Source: CAD feature listing. Evaluate the final solid. Frame: model axes, mm. Face numbers are marked on the shaded views. A direction names the side the tool comes from. Give positions to 0.01 mm unless a question says otherwise; leave off trailing zeros. Order: outer loops, then holes, each group sorted by start corner. A loop starts at its lowest first (then second) coordinate and runs counter-clockwise, first axis right, second up. Notation, with made-up numbers: M 12,45.25 L 57,45.25 A19 cw 57,55.25 Z; hole C -32.75,67 d5. An arc over 180 degrees is marked long. Return JSON: item names as keys, results as strings.
from build123d import *

# Parameters (mm, degrees)
CONE_ROLL_ANGLE        = 90
CYLINDER_R             = 1
CYLINDER_DEPTH         = 3
CYLINDER_ROLL_ANGLE    = 90
CYLINDER005_R          = 3.5
CYLINDER005_DEPTH      = 3
CYLINDER005_ROLL_ANGLE = 90
BOX_W                  = 1
BOX_H                  = 10
BOX_DEPTH              = 10
BOX002_W               = 13
BOX002_H               = 5
BOX002_DEPTH           = 13
CYLINDER002_R          = 2.4
CYLINDER002_DEPTH      = 13
CYLINDER002_ROLL_ANGLE = 90


with BuildPart() as screw_guide:
    # Cone → Cone (revolve)
    with BuildSketch(Plane.XZ):
        Polygon((0, 0), (0.5, 0), (1.5, 7), (0, 7), align=None)
    revolve(axis=Axis((0, 0, 0), (0, 0, 1)))


with BuildPart() as screw_guide_1:
    # Cone roll: moved
    add(screw_guide.part.rotate(Axis((0, 0, 0), (1, 0, 0)), CONE_ROLL_ANGLE))


with BuildPart() as screw_guide_2:
    # Cone placement: moved
    add(screw_guide_1.part.moved(Location((18, 69, 6))))


with BuildPart() as hole:
    # Cylinder → Cylinder (new body)
    with BuildSketch(Plane.XY):
        Circle(CYLINDER_R)
    extrude(amount=CYLINDER_DEPTH)


with BuildPart() as hole_1:
    # Cylinder roll: moved
    add(hole.part.rotate(Axis((0, 0, 0), (1, 0, 0)), CYLINDER_ROLL_ANGLE))


with BuildPart() as hole_2:
    # Cylinder placement: moved
    add(hole_1.part.moved(Location((18, 62, 6))))


with BuildPart() as screw_head_seat:
    # Cylinder005 → Cylinder005 (new body)
    with BuildSketch(Plane.XY):
        Circle(CYLINDER005_R)
    extrude(amount=CYLINDER005_DEPTH)


with BuildPart() as screw_head_seat_1:
    # Cylinder005 roll: moved
    add(screw_head_seat.part.rotate(Axis((0, 0, 0), (1, 0, 0)), CYLINDER005_ROLL_ANGLE))


with BuildPart() as screw_head_seat_2:
    # Cylinder005 placement: moved
    add(screw_head_seat_1.part.moved(Location((18, 59, 6))))


with BuildPart() as hole_and_cut:
    # Box → Box (new body)
    with BuildSketch(Plane(origin=(17.5, 62, 1), x_dir=(1, 0, 0), z_dir=(0, 0, 1))):
        with Locations((0.5, 5)):
            Rectangle(BOX_W, BOX_H)
    extrude(amount=BOX_DEPTH)

    # Fusion: union screw guide, hole, screw head seat
    add(screw_guide_2.part)
    add(hole_2.part)
    add(screw_head_seat_2.part)


with BuildPart() as squared_washer:
    # Box002 → Box002 (new body)
    with BuildSketch(Plane(origin=(11.5, 56, -0.5), x_dir=(1, 0, 0), z_dir=(0, 0, 1))):
        with Locations((6.5, 2.5)):
            Rectangle(BOX002_W, BOX002_H)
    extrude(amount=BOX002_DEPTH)


with BuildPart() as anchor_with_hole_and_cut:
    # Cylinder002 → Cylinder002 (new body)
    with BuildSketch(Plane.XY):
        Circle(CYLINDER002_R)
    extrude(amount=CYLINDER002_DEPTH)


with BuildPart() as anchor_with_hole_and_cut_1:
    # Cylinder002 roll: moved
    add(anchor_with_hole_and_cut.part.rotate(Axis((0, 0, 0), (1, 0, 0)), CYLINDER002_ROLL_ANGLE))


with BuildPart() as anchor_with_hole_and_cut_2:
    # Cylinder002 placement: moved
    add(anchor_with_hole_and_cut_1.part.moved(Location((18, 72, 6))))

    # Fusion001: union squared washer
    add(squared_washer.part)

    # Cut: cut hole and cut
    add(hole_and_cut.part, mode=Mode.SUBTRACT)


solid = anchor_with_hole_and_cut_2.part
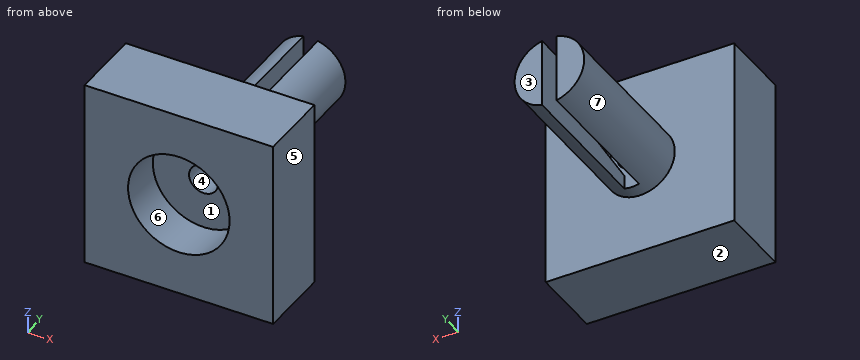
1. Ray query, probe 1 along Z at (x, y) = (18, 56.9); probe 2 along Z at (x, y) = (18, 59.85); probe 3 along Y at (x, z) = (15, 8). Return the intervals inside material, ascending.
Evaluation:
{"probe 1": "z = -0.5 to 2.5, 9.5 to 12.5", "probe 2": "z = -0.5 to 5, 7 to 12.5", "probe 3": "y = 56 to 61"}
2. First-contact query: pin 1 (2.5 mm diameter, centred on y = 67.5, z = 5, fed in from -X); pin 2 (4 mm diameter, centred on y = 67.5, z = 6.5, fed in from +X). Flat tips, straight axial feed; report the tip coordinate or a pass-through.
Evaluation:
{"pin 1": "stops at x = 15.6", "pin 2": "stops at x = 20.4"}
3. Section query A-A (x = 18). Return loops of the section in (y, z).
Evaluation:
{"outline": "M 56,-0.5 L 61,-0.5 L 61,3.6 L 62,3.6 L 62,5 L 59,5 L 59,2.5 L 56,2.5 Z; M 56,9.5 L 59,9.5 L 59,7 L 62,7 L 62,8.4 L 61,8.4 L 61,12.5 L 56,12.5 Z"}
4. Section query C-C (y = 63.5). Return loops of the section in (x, z), then the cut area to 3 significant figures.
Evaluation:
{"outline": "M 17.5,3.65 L 17.5,4.82 A1.29 cw 17.5,7.18 L 17.5,8.35 A2.4 ccw Z; M 18.5,3.65 A2.4 ccw 18.5,8.35 L 18.5,7.18 A1.29 cw 18.5,4.82 Z", "area": "10.6 mm^2"}
5. Section query D-D (y = 58.5). Return loops of the section in (x, z), then the cut area to 3 significant figures.
Evaluation:
{"outline": "M 11.5,-0.5 L 24.5,-0.5 L 24.5,12.5 L 11.5,12.5 Z; hole C 18,6 d7", "area": "131 mm^2"}
6. Section query B-B (z = 6). Return loops of the section in (x, y), then the cut area to 3 significant figures.
Evaluation:
{"outline": "M 11.5,56 L 14.5,56 L 14.5,59 L 17,59 L 17,62 L 16.5,62 L 17.5,69 L 17.5,72 L 15.6,72 L 15.6,61 L 11.5,61 Z; M 18.5,69 L 19.5,62 L 19,62 L 19,59 L 21.5,59 L 21.5,56 L 24.5,56 L 24.5,61 L 20.4,61 L 20.4,72 L 18.5,72 Z", "area": "73.8 mm^2"}
7. Draft query along Z for the marked faces 1, 2, 3 and 4. Return one class per face: pulls with the +Z half, pulls with the -Z half, needs draft (parallel to the pull), parting line crosses it, or undercut.
Evaluation:
{"face 1": "undercut", "face 2": "pulls with the -Z half", "face 3": "needs draft", "face 4": "undercut"}
8. Set-up query: the marked faces 5, 6 and 7. Return all of +Z, -Z, +X, -X, +Y, -Y with unobstructed straight access to the full face (end or side cutting, diameter ignored); none if empty.
Evaluation:
{"face 5": "+Z, -Z, +X, +Y, -Y", "face 6": "-Y", "face 7": "+Y"}
